Geometry: final body of the model. Coordinates: model frame, mm. A direction names the side the tool comes from. Coordinates: 2 decimals unless noted, no trailing zeros. Order: outer loops, then holes, each group sorted by start corner. A loop starts at its lowest first (then second) coordinate and runs counter-clockwise, first axis right, second up. Notation, with made-up numbers: (46, -7) - (102, -7) arc R25 cw to (102, 28) - close; hole circle Ø1 at (60.25, -35). An arc over 180 degrees is marked (long way). Use a Markdown table: item, result. Add a question column.
```python
from build123d import *

# Parameters (mm, degrees)
F0_W     = 3.175
F0_H     = 3.175
F1_DEPTH = 3.175
F2_R     = 0.396875


with BuildPart() as f1:
    # F0 (on Top) → F1 (new body)
    with BuildSketch(Plane.XY):
        with BuildLine():
            ThreePointArc((1.5875, 3.96875), (1.3550160076, 4.5300160076), (0.79375, 4.7625))
            Line((0.79375, 4.7625), (-0.79375, 4.7625))
            ThreePointArc((-0.79375, 4.7625), (-1.3550160076, 4.5300160076), (-1.5875, 3.96875))
            Line((-1.5875, 3.96875), (-1.5875, 1.5875))
            Line((-1.5875, 1.5875), (1.5875, 1.5875))
            Line((1.5875, 1.5875), (1.5875, 3.96875))
        make_face()
        with BuildLine():
            Line((3.96875, 1.5875), (1.5875, 1.5875))
            Line((1.5875, 1.5875), (1.5875, -1.5875))
            Line((1.5875, -1.5875), (3.96875, -1.5875))
            ThreePointArc((3.96875, -1.5875), (4.5300160076, -1.3550160076), (4.7625, -0.79375))
            Line((4.7625, -0.79375), (4.7625, 0.79375))
            ThreePointArc((4.7625, 0.79375), (4.5300160076, 1.3550160076), (3.96875, 1.5875))
        make_face()
        Rectangle(F0_W, F0_H)
        with BuildLine():
            Line((-1.5875, -1.5875), (-1.5875, 1.5875))
            Line((-1.5875, 1.5875), (-3.96875, 1.5875))
            ThreePointArc((-3.96875, 1.5875), (-4.5300160076, 1.3550160076), (-4.7625, 0.79375))
            Line((-4.7625, 0.79375), (-4.7625, -0.79375))
            ThreePointArc((-4.7625, -0.79375), (-4.5300160076, -1.3550160076), (-3.96875, -1.5875))
            Line((-3.96875, -1.5875), (-1.5875, -1.5875))
        make_face()
        with BuildLine():
            Line((1.5875, -3.96875), (1.5875, -1.5875))
            Line((1.5875, -1.5875), (-1.5875, -1.5875))
            Line((-1.5875, -1.5875), (-1.5875, -3.96875))
            ThreePointArc((-1.5875, -3.96875), (-1.3550160076, -4.5300160076), (-0.79375, -4.7625))
            Line((-0.79375, -4.7625), (0.79375, -4.7625))
            ThreePointArc((0.79375, -4.7625), (1.3550160076, -4.5300160076), (1.5875, -3.96875))
        make_face()
    extrude(amount=F1_DEPTH)

    # F2
    f2_edges = [f1.edges().sort_by_distance(p)[0] for p in [
        (1.355016, 4.530016, 3.175),
        (0, 4.7625, 3.175),
        (-1.355016, 4.530016, 3.175),
        (-1.5875, 2.778125, 3.175),
        (-2.778125, 1.5875, 3.175),
        (-4.530016, 1.355016, 3.175),
        (-4.7625, 0, 3.175),
        (-4.530016, -1.355016, 3.175),
        (-2.778125, -1.5875, 3.175),
        (-1.5875, -2.778125, 3.175),
        (-1.355016, -4.530016, 3.175),
        (0, -4.7625, 3.175),
        (1.355016, -4.530016, 3.175),
        (1.5875, -2.778125, 3.175),
        (2.778125, -1.5875, 3.175),
        (4.530016, -1.355016, 3.175),
        (4.7625, 0, 3.175),
        (4.530016, 1.355016, 3.175),
        (2.778125, 1.5875, 3.175),
        (1.5875, 2.778125, 3.175),
        (1.355016, 4.530016, 0),
        (0, 4.7625, 0),
        (-1.355016, 4.530016, 0),
        (-1.5875, 2.778125, 0),
        (-2.778125, 1.5875, 0),
        (-4.530016, 1.355016, 0),
        (-4.7625, 0, 0),
        (-4.530016, -1.355016, 0),
        (-2.778125, -1.5875, 0),
        (-1.5875, -2.778125, 0),
        (-1.355016, -4.530016, 0),
        (0, -4.7625, 0),
        (1.355016, -4.530016, 0),
        (1.5875, -2.778125, 0),
        (2.778125, -1.5875, 0),
        (4.530016, -1.355016, 0),
        (4.7625, 0, 0),
        (4.530016, 1.355016, 0),
        (2.778125, 1.5875, 0),
        (1.5875, 2.778125, 0),
    ]]
    fillet(f2_edges, radius=F2_R)


solid = f1.part
```
1) First-contact query: pin 1 (0.7 mm diameter, centred on x = -3, z = 1, fed in from +Y); pin 2 (1.9 mm diameter, centred on y = 3, z = 1.5, fed in from +X); pin 3 (1.2 mm diameter, centred on x = -2.5, z = 1.5, fed in from -Y). Flat tips, straight axial feed; report the tip coordinate or a pass-through.
2) Access query for faces 1 (the flat face through (1.588, 3, 2)), 2 (the flat face through (-3, -1.588, 2)), 3 (the flat face through (1.588, -3, 2)). Directions: +Z, -Z, +X, -X, +Y, -Y. A direction counts if a zero-diameter tool reaches every point of the face in a straight line with its end or side. Return the directions, or none.
3) Line query: line 1 (X direction, y = 3.5, z = 2.2); line 2 (Y direction, x = -3.75, z = 0.35); line 3 (Y direction, x = -4.25, z = 1.2). Output: solid intervals per line, ascending. Write a range as from..to.
4) Section query A-A (y = -3.25). Return the cut outline in (x, z) (1 decimal).
5) Section query B-B (z = 1.8). Return the cut outline in (x, y).
From the geometry:
| question | item | result |
|---|---|---|
| 1 | pin 1 | stops at y = 1.59 |
| 1 | pin 2 | stops at x = 1.59 |
| 1 | pin 3 | stops at y = -1.59 |
| 2 | face 1 | +Z, -Z, +X, +Y |
| 2 | face 2 | +Z, -Z, -X, -Y |
| 2 | face 3 | +Z, -Z, +X, -Y |
| 3 | line 1 | x = -1.59..1.59 |
| 3 | line 2 | y = -1.58..1.58 |
| 3 | line 3 | y = -1.54..1.54 |
| 4 | outline | (-1.6, 0.4) arc R0.4 ccw to (-1.2, 0) - (1.2, 0) arc R0.4 ccw to (1.6, 0.4) - (1.6, 2.8) arc R0.4 ccw to (1.2, 3.2) - (-1.2, 3.2) arc R0.4 ccw to (-1.6, 2.8) - close |
| 5 | outline | (-4.76, -0.79) arc R0.79 ccw to (-3.97, -1.59) - (-1.59, -1.59) - (-1.59, -3.97) arc R0.79 ccw to (-0.79, -4.76) - (0.79, -4.76) arc R0.79 ccw to (1.59, -3.97) - (1.59, -1.59) - (3.97, -1.59) arc R0.79 ccw to (4.76, -0.79) - (4.76, 0.79) arc R0.79 ccw to (3.97, 1.59) - (1.59, 1.59) - (1.59, 3.97) arc R0.79 ccw to (0.79, 4.76) - (-0.79, 4.76) arc R0.79 ccw to (-1.59, 3.97) - (-1.59, 1.59) - (-3.97, 1.59) arc R0.79 ccw to (-4.76, 0.79) - close |
